Autodesk Inventor part; units mm, degrees
ref_plane "YZ Plane" through (0, 0, 0) normal (1, 0, 0) x (0, 1, 0)
ref_plane "XZ Plane" through (0, 0, 0) normal (0, 1, 0) x (-1, 0, 0)
ref_plane "XY Plane" through (0, 0, 0) normal (0, 0, 1) x (1, 0, 0)
sketch "Boceto1" plane through (0, 0, 0) normal (0, 1, 0) x (-1, 0, 0)
  arc A0 (-18, 72.808) -> (20, 72.2842) centre (0, 0) ccw
  line L0 (-18, 72.808) -> (-18, 72.2842)
  line L1 (-11, 25) -> (13, 25)
  line L2 (55, 8) -> (40, 8)
  line L3 (40, 8) -> (40, -42)
  line L4 (40, -42) -> (55, -42)
  line L5 (55, -42) -> (55, 8)
  line L6 (-40, 8) -> (-55, 8)
  line L7 (-55, 8) -> (-55, -42)
  line L8 (-55, -42) -> (-40, -42)
  line L9 (-40, -42) -> (-40, 8)
  line L10 (20, 72.2842) -> (13, 72.2842)
  line L11 (13, 72.2842) -> (13, 25)
  line L12 (-18, 72.808) -> (-11, 72.808)
  line L13 (-11, 72.808) -> (-11, 25)
  line L14 (-18, 72.2842) -> (-18, 72.808)
  dimension "d0" = 150
  dimension "d2" = 18
  dimension "d3" = 25
  dimension "d4" = 15
  dimension "d5" = 50
  dimension "d6" = 15
  dimension "d7" = 50
  dimension "d8" = 40
  dimension "d9" = 40
  dimension "d63" = 8
  dimension "d64" = 8
extrude "Extrusión1" add sketch "Boceto1" along normal blind 2
sketch "Boceto8" plane through (0, 0, 0) normal (0, 1, 0) x (-1, 0, 0)
  line L0 (59.5508, 67.2842) -> (-59.748, 67.2842)
  line L1 (-59.748, 67.2842) -> (-59.748, 82.2842)
  line L2 (-59.748, 82.2842) -> (59.5508, 82.2842)
  line L3 (59.5508, 82.2842) -> (59.5508, 67.2842)
  line L4 (13, 72.2842) -> (20, 72.2842)
  point P0 (0, 0)
  dimension "d67" = 15
  dimension "d71" = 5
extrude "Extrusión8" cut sketch "Boceto8" along normal mid plane 70
properties part number "Cuerpo" material "Polímero reforzado con fibra de carbono"
Work out the finished part from the listing and answer in its coordinate system (mm). Coordinates: 2 decimals unless noted, no trailing zeros. Write each loop counter-clockwise with the first axis right and the second up, starting at its lowest first coordinate (ties: lowest second). Pieces come first, ordered by that corner, then holes. Notation, with made-up numbers: M 9.5,8 L 38.5,8 A17 cw 38.5,20 Z; hole C -0.5,-12 d11. An arc over 180 degrees is marked long. Answer as CSV lines item,"result". Start each with the question number.
Item 1: Section B-B on y = 0.6 is taken. Write down the section's boundary in (x, z), and give its area (3 significant figures).
Item 2: Section C-C on z = -19.5 is taken. Write down the section's boundary in (x, y).
Item 3: Section A-A on x = -52 is taken. Write down the section's boundary in (y, z), and give its area (3 significant figures).
Item 4: Consider L1, parallel to X at y = 0.95, z = 4; L2, parallel to Z at x = 51, y = 1.95; L3, parallel to X at y = 1.75, z = -40.5. Determine where each line is inside the solid, lowest interval first.
Item 5: Section D-D on z = 28.5 is taken. Write down the section's boundary in (x, y), and give its area (3 significant figures).
Item 6: Flat-ended cylindrical pins translate along their axes: P1, Ø1, axis at y = 1, z = -25, coming from the +X side; P2, Ø1, axis at x = -50, y = 0.5, coming from the -Z side (3 decimals); P3, Ø1, axis at y = 1.5, z = -5.5, coming from the +X side. Find the tip coordinate at first contact, or state that the pin passes through.
Checks:
1,outline,"M -33.13,67.28 A75 ccw long 33.13,67.28 L 11,67.28 L 11,25 L -13,25 L -13,67.28 Z; hole M -55,-42 L -40,-42 L -40,8 L -55,8 Z; hole M 40,-42 L 55,-42 L 55,8 L 40,8 Z"
1,area,"14,800 mm²"
2,outline,"M -72.42,0 L -55,0 L -55,2 L -72.42,2 Z; M -40,0 L 40,0 L 40,2 L -40,2 Z; M 55,0 L 72.42,0 L 72.42,2 L 55,2 Z"
3,outline,"M 0,-54.05 L 2,-54.05 L 2,-42 L 0,-42 Z; M 0,8 L 2,8 L 2,54.05 L 0,54.05 Z"
3,area,"116 mm²"
4,L1,"x = -74.89 to -55, -40 to 40, 55 to 74.89"
4,L2,"z = -54.99 to -42, 8 to 54.99"
4,L3,"x = -63.12 to -55, -40 to 40, 55 to 63.12"
5,outline,"M -69.37,0 L -13,0 L -13,2 L -69.37,2 Z; M 11,0 L 69.37,0 L 69.37,2 L 11,2 Z"
5,area,"229 mm²"
6,P1,"stops at x = 70.89"
6,P2,"stops at z = -56.345"
6,P3,"stops at x = 74.83"
